from build123d import *

# Parameters (mm, degrees)
BOSS_EXTRUDE1_DEPTH = 10
CHAMFER1_SIZE       = 1


with BuildPart() as part:
    # Sketch1 → Boss-Extrude1 (new body)
    with BuildSketch(Plane.XY):
        Polygon((-14.285879212, 0), (-14.285879212, -10), (-5.285879212, -10), (-5.285879212, -18), (6.714120788, -18), (6.714120788, -10), (15.714120788, -10), (15.714120788, 0), (20.714120788, 0), (20.714120788, -21), (-19.285879212, -21), (-19.285879212, 0), align=None)
    extrude(amount=BOSS_EXTRUDE1_DEPTH)

    # Chamfer1
    chamfer1_edges = [part.edges().sort_by_distance(p)[0] for p in [
        (20.714120788, -10.5, 0),
        (0.714120788, -21, 0),
        (11.214120788, -10, 10),
        (-19.285879212, -10.5, 0),
        (-16.785879212, 0, 0),
        (-14.285879212, -5, 0),
        (-9.785879212, -10, 0),
        (-5.285879212, -14, 0),
        (0.714120788, -18, 0),
        (6.714120788, -14, 0),
        (11.214120788, -10, 0),
        (15.714120788, -5, 0),
        (18.214120788, 0, 0),
        (6.714120788, -14, 10),
        (0.714120788, -18, 10),
        (-5.285879212, -14, 10),
        (-9.785879212, -10, 10),
        (-14.285879212, -5, 10),
        (-16.785879212, 0, 10),
        (-19.285879212, -10.5, 10),
        (0.714120788, -21, 10),
        (20.714120788, -10.5, 10),
        (18.214120788, 0, 10),
        (15.714120788, -5, 10),
    ]]
    chamfer(chamfer1_edges, length=CHAMFER1_SIZE)


solid = part.part
Source: CAD feature listing. Evaluate the final solid. Frame: model axes, mm. A direction names the side the tool comes from. Coordinates: 2 decimals unless noted, no trailing zeros. Loops run counter-clockwise (first coordinate to the right, second up) from the corner with the lowest first, then second, coordinate; pieces in that order, holes last. Notation, with made-up numbers: (42.25, -18) - (72.25, -18) arc R28 ccw to (72.25, 11) - close; hole circle Ø11 at (-28.75, -7). An arc over 180 degrees is marked (long way). One line per item, written item: value. Start each with the question number.
1. Section D-D (y = -16.75). Return the cut outline in (x, z), and give its area (3 significant figures).
2. Mould query, pull axis X, two halves, no side actions, for faces 1 (the flat face through (-19.286, -11, 5)), 2 (the flat face through (18, 0, 5)), 3 (the flat face through (16.221, -5.577, 9.507)), 4 (the flat face through (20.714, -10, 5)). Classes: pulls with the +X half, pulls with the -X half, needs draft (parallel to the pull), parting line crosses it, or undercut.
3. Contact query for flat-ended pins moving along their axis: P1, Ø1.5, axis at x = -4, y = -9.5, coming from the +Z side; P2, Ø2.5, axis at x = 13, z = 5, coming from the +Y side; P3, Ø4, axis at x = -1, z = 6, coming from the +Y side; P4, Ø1.5, axis at x = -11.5, y = -10, coming from the -Z side. Output: stop coordinate, or through.
4. Ray query, L1, parallel to X at y = -10.25, z = 7.25; L2, parallel to X at y = -5.75, z = 1.75; L3, parallel to Y at x = -10, z = 3.25. Return the intervals inside material, ascending.
5. Set-up query: faces 5 (the flat face through (7.221, -14.563, 9.507)), 6 (the flat face through (15.714, -5, 5)), 7 (the flat face through (18.2, -0.5, 0.5)), 8 (the flat face through (0.6, -18.5, 0.5)), 9 (the flat face through (-18.779, -10.647, 9.507)). Return all of +Z, -Z, +X, -X, +Y, -Y with unobstructed straight access to the full face (end or side cutting, diameter ignored); none if empty.
6. Section C-C (z = 8.5). Return the cut outline in (x, y).
7. Section B-B (x = -11). Return the cut outline in (y, z).
8. Section A-A (y = -7). Return the cut outline in (x, z).
Verdict:
1. outline: (-19.29, 1) - (-18.29, 0) - (-6.29, 0) - (-5.29, 1) - (-5.29, 9) - (-6.29, 10) - (-18.29, 10) - (-19.29, 9) - close; (6.71, 1) - (7.71, 0) - (19.71, 0) - (20.71, 1) - (20.71, 9) - (19.71, 10) - (7.71, 10) - (6.71, 9) - close
1. area: 276 mm2
2. face 1: pulls with the -X half
2. face 2: needs draft
2. face 3: undercut
2. face 4: pulls with the +X half
3. P1: passes through
3. P2: stops at y = -10
3. P3: stops at y = -18
3. P4: stops at z = 0.25
4. L1: x = -19.29 to -5.29, 6.71 to 20.71
4. L2: x = -19.29 to -14.29, 15.71 to 20.71
4. L3: y = -21 to -10
5. face 5: +Z, +Y
5. face 6: +Z, -Z, +Y
5. face 7: -Z, +X, -X, +Y
5. face 8: -Z, +Y
5. face 9: +Z, -X, +Y, -Y
6. outline: (-19.29, -21) - (20.71, -21) - (20.71, 0) - (15.71, 0) - (15.71, -10) - (6.71, -10) - (6.71, -18) - (-5.29, -18) - (-5.29, -10) - (-14.29, -10) - (-14.29, 0) - (-19.29, 0) - close
7. outline: (-21, 1) - (-20, 0) - (-11, 0) - (-10, 1) - (-10, 9) - (-11, 10) - (-20, 10) - (-21, 9) - close
8. outline: (-19.29, 1) - (-18.29, 0) - (-15.29, 0) - (-14.29, 1) - (-14.29, 9) - (-15.29, 10) - (-18.29, 10) - (-19.29, 9) - close; (15.71, 1) - (16.71, 0) - (19.71, 0) - (20.71, 1) - (20.71, 9) - (19.71, 10) - (16.71, 10) - (15.71, 9) - close
